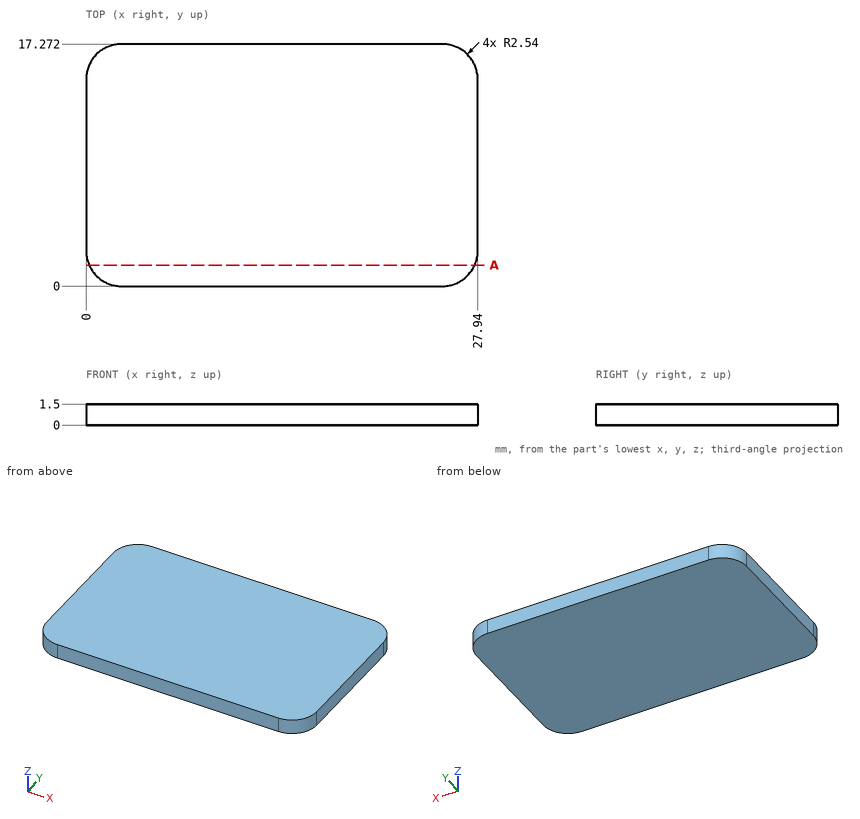
Here's the drawing with two shaded views (mm, measured from the low corner). I have some questions. Coordinates: 2 decimals unless noted, no trailing zeros. Loops run counter-clockwise (first coordinate to the right, second up) from the corner with the lowest first, then second, coordinate; pieces in that order, holes last. Notation, with made-up numbers: (41, 2.5) -> (75, 2.5) arc R24 cw to (75, 25.5) -> close; hole circle Ø5 at (46.5, -27.75). An arc over 180 degrees is marked (long way). Use one line per item in the form item = value. Start each with the question number.
(1) Will this pin go through, and if not, where does the flat tip stop? pin 1 (5 mm diameter, centred on x = 12, y = 10.5, fed in from -Z).
(2) If we section it at A-A (y = 1.5): Please give me the cut outline in (x, z), then the cut area to 3 significant figures.
(3) Please list where these lines run through material, in increasing order: line 1 along X through (y, z) = (16.25, 0.9); line 2 along X through (y, z) = (0.5, 0.15).
Verdict:
q1.pin_1 = 0
q2.outline = (0.22, 0) -> (27.72, 0) -> (27.72, 1.5) -> (0.22, 1.5) -> close
q2.area = 41.2 mm²
q3.line_1 = 0.5 to 27.44
q3.line_2 = 1.03 to 26.91
